Check sheet for the drawn part. Datum: minimum x, y, z corner. Units: mm. A direction names the side the tool comes from. Give positions to 0.01 mm unless a question says otherwise; leave off trailing zeros. Order: outer loops, then holes, each group sorted by start corner. A loop starts at its lowest first (then second) coordinate and runs counter-clockwise, first axis right, second up. Notation, with made-up numbers: (16, 80) -> (27, 80) arc R17 cw to (27, 88) -> close; hole circle Ø4 at (-39.75, 18). An arc over 180 degrees is marked (long way). Return JSON: item names as keys, results as strings. Group by question number.
(1) Cross-section at D-D on y = 8.5. Enter the section's corners in (x, z).
(2) Depth check by flat-ended pin: pin 1 Ø4.5 at (y, z) = (5.5, 28.5) entering from -X; pin 2 Ø10 at (x, z) = (9.5, 9) entering from -Y; pin 3 Ø1.5 at (x, y) = (35, 7.5) entering from -Z; pin 4 Ø4 at (x, y) = (31, 5) entering from +Z. Enter the tip coordinate at first touch or a pass-through.
(3) Tool access check on the marked faces 1, 2 and 3. Record the directions out of +Z, -Z, +X, -X, +Y, -Y that give a thin tool (end or side, any length) a straight path to the whole face; none if there is none.
(4) Release check for a two-part mould opening along Z. For the marked faces 4, 5 and 6 record: pulls with the +Z half, pulls with the -Z half, needs draft (parallel to the pull), parting line crosses it, or undercut.
(5) Cross-section at C-C on z = 27.75. Enter the section's corners in (x, y), then the cut area to 3 significant figures.
(6) Cross-section at A-A on z = 21.5. Enter the section's corners in (x, y), then the cut area to 3 significant figures.
(7) Cross-section at B-B on y = 5. Enter the section's corners in (x, z) (3 decimals), then the cut area to 3 significant figures.
(8) Thickness scan on line 1 along Z through (x, y) = (30.75, 12.7); line 2 along X through (y, z) = (12.75, 25); line 3 along Y through (x, z) = (26, 22.5). Record the ranges inside material, lowest first.
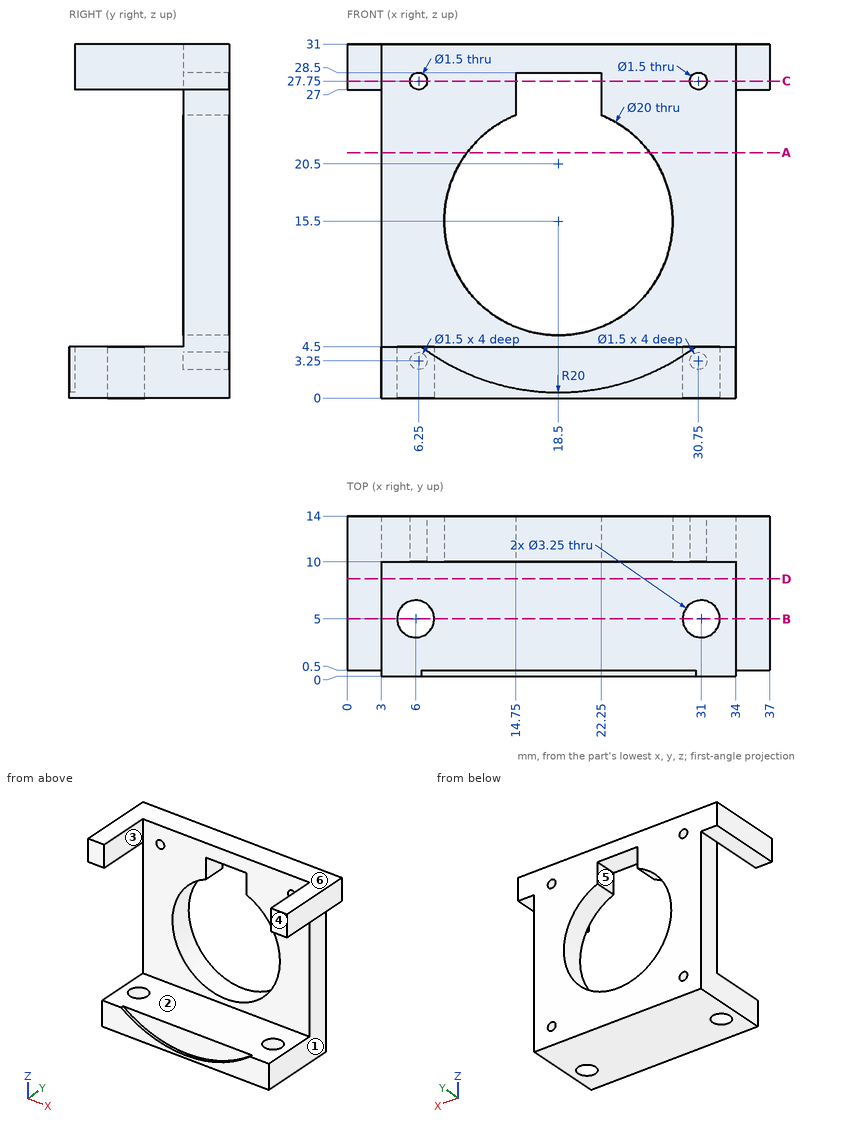
Verdict:
{
 "1": {"outline": "(0, 27) -> (3, 27) -> (3, 31) -> (0, 31) -> close; (3, 0) -> (34, 0) -> (34, 4.5) -> (3, 4.5) -> close; (34, 27) -> (37, 27) -> (37, 31) -> (34, 31) -> close"},
 "2": {"pin 1": "x = 0", "pin 2": "y = 0.5", "pin 3": "z = 27", "pin 4": "z = 4.5"},
 "3": {"face 1": "-Z, +X, +Y, -Y", "face 2": "+Z, +X, -X, -Y", "face 3": "+Z, -Y"},
 "4": {"face 4": "needs draft", "face 5": "undercut", "face 6": "pulls with the +Z half"},
 "5": {"outline": "(0, 0.5) -> (3, 0.5) -> (3, 10) -> (5.5, 10) -> (5.5, 14) -> (0, 14) -> close; (7, 10) -> (14.75, 10) -> (14.75, 14) -> (7, 14) -> close; (22.25, 10) -> (30, 10) -> (30, 14) -> (22.25, 14) -> close; (31.5, 10) -> (34, 10) -> (34, 0.5) -> (37, 0.5) -> (37, 14) -> (31.5, 14) -> close", "area": "163 mm²"},
 "6": {"outline": "(3, 10) -> (10.5, 10) -> (10.5, 14) -> (3, 14) -> close; (26.5, 10) -> (34, 10) -> (34, 14) -> (26.5, 14) -> close", "area": "60.0 mm²"},
 "7": {"outline": "(0, 27) -> (3, 27) -> (3, 31) -> (0, 31) -> close; (3, 0) -> (4.375, 0) -> (4.375, 4.5) -> (3, 4.5) -> close; (7.625, 0) -> (29.375, 0) -> (29.375, 4.5) -> (7.625, 4.5) -> close; (32.625, 0) -> (34, 0) -> (34, 4.5) -> (32.625, 4.5) -> close; (34, 27) -> (37, 27) -> (37, 31) -> (34, 31) -> close", "area": "134 mm²"},
 "8": {"line 1": "0 to 2.5, 4 to 27, 28.5 to 31", "line 2": "3 to 14.75, 22.25 to 34", "line 3": "10 to 14"}
}
